Geometry: final body of the model. Coordinates: model frame, mm. A direction names the side the tool comes from. Give positions to 0.01 mm unless a question says otherwise; leave off trailing zeros. Write each loop counter-clockwise with the first axis right and the second up, starting at its lowest first coordinate (ties: lowest second). Pieces come first, ordered by that corner, then holes. Notation, with made-up numbers: M 8.5,51.25 L 33.5,51.25 A5 cw 33.5,60.25 Z; hole C 52,-14 d2. An arc over 180 degrees is marked long. Answer as a JSON object with one key per item and string values.
from build123d import *

# Parameters (mm, degrees)
F0_R     = 2.5019
F1_DEPTH = 3.175
F2_W     = 12.7
F2_H     = 3.175
F2_W_2   = 74.0918
F3_DEPTH = 9.525
F4_W     = 12.7
F4_H     = 3.175
F5_W     = 12.7
F5_H     = 3.175
F6_DEPTH = 3.175
F7_W     = 74.0918
F7_H     = 3.175
F8_DEPTH = 3.175
F9_R     = 3.17499


# Not quite as in the source:
# - a fillet or chamfer is up to 0.001 mm smaller than in the source, because OpenCascade refuses the exact size
# - a feature names something its author has since deleted; it is built from what else it names


with BuildPart() as f1:
    # F0 (on Front) → F1 (new body)
    with BuildSketch(Plane.XZ):
        Polygon((49.7459, 20.6375), (-49.7459, 20.6375), (-49.7459, -20.6375), (-37.0459, -20.6375), (-37.0459, 7.9375), (37.0459, 7.9375), (37.0459, -20.6375), (49.7459, -20.6375), align=None)
        with Locations((-42.9895, 13.8811)):
            Circle(F0_R, mode=Mode.SUBTRACT)
        with Locations((42.9895, 13.8811)):
            Circle(F0_R, mode=Mode.SUBTRACT)
    extrude(amount=F1_DEPTH)

    # F2 (on face) → F3 (join)
    with BuildSketch(Plane.XZ.offset(3.175)):
        with Locations((-43.3959, -19.05)):
            Rectangle(F2_W, F2_H)
        with Locations((0, 9.525)):
            Rectangle(F2_W_2, F2_H)
        with Locations((43.3959, -19.05)):
            Rectangle(F2_W, F2_H)
    extrude(amount=F3_DEPTH)

    # F4 (on face) + F5 (on face) → F6 (join)
    with BuildSketch(Plane.XY.offset(-17.4625)):
        with Locations((-43.3959, -11.1125)):
            Rectangle(F4_W, F4_H)
    with BuildSketch(Plane.XY.offset(-17.4625)):
        with Locations((43.3959, -11.1125)):
            Rectangle(F5_W, F5_H)
    extrude(amount=F6_DEPTH)

    # F7 (on face) → F8 (join)
    with BuildSketch(Plane(origin=(0, 0, 7.9375), x_dir=(1, 0, 0), z_dir=(0, 0, -1))):
        with Locations((0, 11.1125)):
            Rectangle(F7_W, F7_H)
    extrude(amount=F8_DEPTH)

    # F9 (radius 3.175 in the source; OpenCascade refuses exactly that, so slightly less here)
    f9_edges = [f1.edges().sort_by_distance(p)[0] for p in [
        (-49.7459, -1.5875, 20.6375),
        (-49.7459, -6.35, -20.6375),
        (-49.7459, -11.1125, -14.2875),
        (-37.0459, -7.9375, 11.1125),
        (-37.0459, -11.1125, 4.7625),
        (-37.0459, -11.1125, -14.2875),
        (-37.0459, -6.35, -20.6375),
        (49.7459, -1.5875, 20.6375),
        (49.7459, -6.35, -20.6375),
        (37.0459, -7.9375, 11.1125),
        (37.0459, -11.1125, 4.7625),
        (37.0459, -11.1125, -14.2875),
        (37.0459, -6.35, -20.6375),
        (49.7459, -11.1125, -14.2875),
    ]]
    fillet(f9_edges, radius=F9_R)


solid = f1.part
1) Set-up query: faces 1 (the flat face through (43, -12.7, -17)), 2 (the cylindrical face through (-48.8, -11.1, -15.2)), 3 (the flat face through (43, -6, -17.463)). Return all of +Z, -Z, +X, -X, +Y, -Y with unobstructed straight access to the full face (end or side cutting, diameter ignored); none if empty.
Geometry check:
{"face 1": "+Z, -Z, +X, -X, -Y", "face 2": "+Z, -X, -Y", "face 3": "+Z, +X, -X"}
2) Pull-direction query (Y, two-part tool) for faces 4 (the flat face through (-43, -6, -17.463)), 5 (the flat face through (-1, 0, 9)), 6 (the flat face through (-43, -11, -14.287)); classes: pulls with the +Y half, pulls with the -Y half, needs draft (parallel to the pull), parting line crosses it, or undercut.
Geometry check:
{"face 4": "undercut", "face 5": "pulls with the +Y half", "face 6": "needs draft"}
3) Contact query for flat-ended pins moving along their axis: P1, Ø2.5, axis at x = 43.5, y = -11.5, coming from the +Z side; P2, Ø1.6, axis at x = -6, y = -11.5, coming from the -Z side; P3, Ø1, axis at y = -7, z = 11, coming from the +X side. Output: stop coordinate, or through.
Geometry check:
{"P1": "stops at z = -14.29", "P2": "stops at z = 4.76", "P3": "stops at x = 35.75"}
4) Cut plane C-C on z = 3. Return loops of the section in (x, y) (3 decimals).
Geometry check:
{"outline": "M -49.746,-3.175 L -37.046,-3.175 L -37.046,0 L -49.746,0 Z; M 37.046,-3.175 L 49.746,-3.175 L 49.746,0 L 37.046,0 Z"}
5) Cut plane B-B on x = 31. Return loops of the section in (y, z) (1 decimal).
Geometry check:
{"outline": "M -12.7,4.8 L -9.5,4.8 L -9.5,7.9 L 0,7.9 L 0,20.6 L -3.2,20.6 L -3.2,11.1 L -12.7,11.1 Z"}
6) Line query: line 1 (X direction, y = -1.5, z = -17.5); line 2 (Y direction, x = -23.5, z = 18.5) (3 decimals); line 3 (Z direction, x = -1, y = -11.75). Output: solid intervals per line, ascending. Write a range as from..to.
Geometry check:
{"line 1": "x = -49.75..-37.05, 37.05..49.75", "line 2": "y = -3.175..0", "line 3": "z = 4.76..11.11"}
7) Cut plane D-D on z = 13. Return loops of the section in (x, y) (3 decimals), and give its area (3 significant figures).
Geometry check:
{"outline": "M -49.746,-3.175 L -45.331,-3.175 L -45.331,0 L -49.746,0 Z; M -40.648,-3.175 L 40.648,-3.175 L 40.648,0 L -40.648,0 Z; M 45.331,-3.175 L 49.746,-3.175 L 49.746,0 L 45.331,0 Z", "area": "286 mm2"}
8) Cut plane A-A on y = -11.25. Give the number of separate pieces and of enclosed holes in the cut face, and give its area (3 significant figures).
Geometry check:
{"separate pieces": "3", "enclosed holes": "0", "area": "606 mm2"}
